Source: CAD feature listing. Evaluate the final solid. Frame: model axes, mm. Face numbers are marked on the shaded views. Round coordinates to 2 decimals unless told otherwise and drop trailing zeros. Order: outer loops, then holes, each group sorted by start corner. A loop starts at its lowest first (then second) coordinate and runs counter-clockwise, first axis right, second up. Notation, with made-up numbers: (89, 59) -> (145, 59) arc R27 ccw to (145, 85) -> close; hole circle Ø6 at (7, 22.25). An arc over 180 degrees is marked (long way). Answer as CSV lines item,"result".
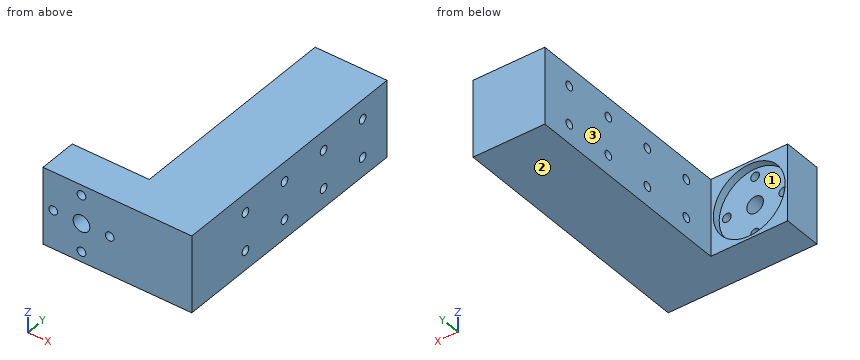
from build123d import *

# Parameters (mm, degrees)
BOSS_EXTRUDE1_DEPTH = 30
SKETCH3_R           = 14
CUT_EXTRUDE1_DEPTH  = 3
SKETCH4_R           = 1.7
SKETCH4_R_2         = 3.25
CUT_EXTRUDE2_DEPTH  = 110.581020254
SKETCH5_R           = 1.7
CUT_EXTRUDE3_DEPTH  = 109.627804912


with BuildPart() as part:
    # Sketch2 → Boss-Extrude1 (new body)
    with BuildSketch(Plane.XY):
        Polygon((0, 0), (0, 15), (30, 15), (30, 100), (58, 100), (58, 0), (30, 0), align=None)
    extrude(amount=BOSS_EXTRUDE1_DEPTH)

    # Sketch3 → Cut-Extrude1 (cut)
    with BuildSketch(Plane(origin=(0, 15, 0), x_dir=(1, 0, 0), z_dir=(0, 1, 0))):
        with Locations(Location((15, -15, 0), (0, 0, 270))):
            Circle(SKETCH3_R)
    extrude(amount=-CUT_EXTRUDE1_DEPTH, mode=Mode.SUBTRACT)

    # Sketch4 → Cut-Extrude2 (cut, through all)
    with BuildSketch(Plane(origin=(0, 12, 0), x_dir=(1, 0, 0), z_dir=(0, 1, 0))):
        with Locations(Location((15, -4, 0), (0, 0, 270))):
            Circle(SKETCH4_R)
        with Locations(Location((26, -15, 0), (0, 0, 270))):
            Circle(SKETCH4_R)
        with Locations(Location((15, -26, 0), (0, 0, 270))):
            Circle(SKETCH4_R)
        with Locations(Location((4, -15, 0), (0, 0, 270))):
            Circle(SKETCH4_R)
        with Locations(Location((15, -15, 0), (0, 0, 270))):
            Circle(SKETCH4_R_2)
    extrude(amount=-CUT_EXTRUDE2_DEPTH, mode=Mode.SUBTRACT)

    # Sketch5 → Cut-Extrude3 (cut, through all)
    with BuildSketch(Plane.ZY.offset(-30)):
        with Locations(Location((7.558876463, 27.5, 0), (0, 0, 270))):
            Circle(SKETCH5_R)
        with Locations(Location((7.558876463, 47.5, 0), (0, 0, 270))):
            Circle(SKETCH5_R)
        with Locations(Location((7.558876463, 67.5, 0), (0, 0, 270))):
            Circle(SKETCH5_R)
        with Locations(Location((7.558876463, 87.5, 0), (0, 0, 270))):
            Circle(SKETCH5_R)
        with Locations(Location((22.441123537, 27.5, 0), (0, 0, 90))):
            Circle(SKETCH5_R)
        with Locations(Location((22.441123537, 47.5, 0), (0, 0, 90))):
            Circle(SKETCH5_R)
        with Locations(Location((22.441123537, 67.5, 0), (0, 0, 90))):
            Circle(SKETCH5_R)
        with Locations(Location((22.441123537, 87.5, 0), (0, 0, 90))):
            Circle(SKETCH5_R)
    extrude(amount=-CUT_EXTRUDE3_DEPTH, mode=Mode.SUBTRACT)


solid = part.part
1. Section query A-A on z = 15. Return loops of the section in (x, y), and give its area (3 significant figures).
Results below:
outline,"(0, 0) -> (2.3, 0) -> (2.3, 12) -> (1, 12) -> (1, 15) -> (0, 15) -> close; (5.7, 0) -> (11.75, 0) -> (11.75, 12) -> (5.7, 12) -> close; (18.25, 0) -> (24.3, 0) -> (24.3, 12) -> (18.25, 12) -> close; (27.7, 0) -> (58, 0) -> (58, 100) -> (30, 100) -> (30, 15) -> (29, 15) -> (29, 12) -> (27.7, 12) -> close"
area,"3,010 mm2"
2. Mould query, pull axis Z, two halves, no side actions, for the marked faces 1, 2 and 3. Classes: released by +Z, released by -Z, zero draft, split by the parting line, or undercut.
Results below:
face 1,"undercut"
face 2,"released by -Z"
face 3,"zero draft"
3. Pin query (flat end, axial travel): pin 1 (4 mm diameter, centred on x = 4, z = 15, fed in from +Y); pin 2 (4.5 mm diameter, centred on y = 27.5, z = 7.56, fed in from -X); pin 3 (1.5 mm diameter, centred on x = 45.5, z = 8.5, fed in from -Y); pin 4 (2 mm diameter, centred on x = 9, z = 27, fed in from +Y). Return the tip coordinate at first contact, or that it passes through.
Results below:
pin 1,"y = 12"
pin 2,"x = 30"
pin 3,"y = 0"
pin 4,"y = 15"
4. Section query B-B on x = 15. Return loops of the section in (y, z).
Results below:
outline,"(0, 0) -> (15, 0) -> (15, 1) -> (12, 1) -> (12, 2.3) -> (0, 2.3) -> close; (0, 5.7) -> (12, 5.7) -> (12, 11.75) -> (0, 11.75) -> close; (0, 18.25) -> (12, 18.25) -> (12, 24.3) -> (0, 24.3) -> close; (0, 27.7) -> (12, 27.7) -> (12, 29) -> (15, 29) -> (15, 30) -> (0, 30) -> close"
5. Section query D-D on x = 26. Return loops of the section in (y, z), and give its area (3 significant figures).
Results below:
outline,"(0, 0) -> (15, 0) -> (15, 6.34) -> (12, 6.34) -> (12, 13.3) -> (0, 13.3) -> close; (0, 16.7) -> (12, 16.7) -> (12, 23.66) -> (15, 23.66) -> (15, 30) -> (0, 30) -> close"
area,"357 mm2"
6. Section query C-C on y = 47.5. Return loops of the section in (x, z), and give its area (3 significant figures).
Results below:
outline,"(30, 0) -> (58, 0) -> (58, 5.86) -> (30, 5.86) -> close; (30, 9.26) -> (58, 9.26) -> (58, 20.74) -> (30, 20.74) -> close; (30, 24.14) -> (58, 24.14) -> (58, 30) -> (30, 30) -> close"
area,"650 mm2"
7. Line query: L1, parallel to Z at x = 47.5, y = 47.5; L2, parallel to Y at x = 37, z = 22.25; L3, parallel to X at y = 8.5, z = 15. Output: solid intervals per line, ascending. Write a range as [from, to].
Results below:
L1,"[0, 5.86], [9.26, 20.74], [24.14, 30]"
L2,"[0, 25.81], [29.19, 45.81], [49.19, 65.81], [69.19, 85.81], [89.19, 100]"
L3,"[0, 2.3], [5.7, 11.75], [18.25, 24.3], [27.7, 58]"
